The listing builds one solid part. Answer for the finished solid, in the listing's coordinates (mm). Coordinates: 2 decimals unless noted, no trailing zeros. Loops run counter-clockwise (first coordinate to the right, second up) from the corner with the lowest first, then second, coordinate; pieces in that order, holes last. Notation, with made-up numbers: M 17,-10.5 L 44,-10.5 A16 cw 44,0.5 Z; hole C 19.25,-8.5 d9. An arc over 180 degrees is marked long. Return JSON: item names as keys, results as strings. Group by question number.
1. Straight lines are drawn through the part: L1, parallel to Z at x = 209.5, y = -2.75; L2, parallel to Y at x = 290, z = -7.2. For each, find the intervals that lie inside material, in ascending order. Write a range as from..to.
2. Given P1, Ø3.5, axis at x = 290, y = 0, coming from the +Z side; P2, Ø4, axis at x = 20, y = 0, coming from the -Z side, each flat-ended and moving along its own axis, determine where each tip first touches the part or whether it passes through.
3. Section B-B (z = 1.5) is taken. Write down the section's boundary in (x, y), then the cut area to 3 significant figures.
4. Section A-A (x = 164) is taken. Write down the section's boundary in (y, z), then the cut area to 3 significant figures.
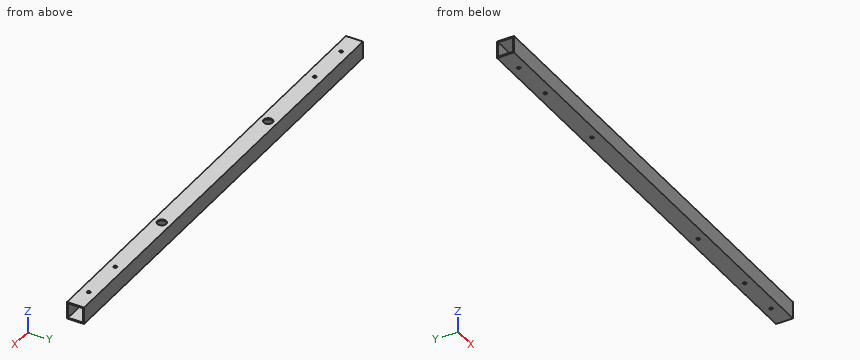
```python
from build123d import *

# Parameters (mm, degrees)
SKETCH_1_W          = 15
SKETCH_1_H          = 15
SKETCH_1_W_2        = 13
SKETCH_1_H_2        = 13
EXTRUDE_1_DEPTH     = 420
SKETCH_2_R          = 1.5
CUT_EXTRUDE_1_DEPTH = 421.334688076
SKETCH_3_R          = 4
CUT_EXTRUDE_2_DEPTH = 10


with BuildPart() as part:
    # 草图1 → 凸台-拉伸1 (new body)
    with BuildSketch(Plane(origin=(0, 0, 0), x_dir=(0, 0, -1), z_dir=(1, 0, 0))):
        Rectangle(SKETCH_1_W, SKETCH_1_H)
        Rectangle(SKETCH_1_W_2, SKETCH_1_H_2, mode=Mode.SUBTRACT)
    extrude(amount=EXTRUDE_1_DEPTH)

    # 草图2 → 切除-拉伸1 (cut, through all)
    with BuildSketch(Plane.XY.offset(7.5)):
        with Locations((20, 0)):
            Circle(SKETCH_2_R)
        with Locations((60, 0)):
            Circle(SKETCH_2_R)
        with Locations((130, 0)):
            Circle(SKETCH_2_R)
        with Locations(Location((290, 0, 0), (0, 0, 270))):
            Circle(SKETCH_2_R)
        with Locations(Location((360, 0, 0), (0, 0, 270))):
            Circle(SKETCH_2_R)
        with Locations(Location((400, 0, 0), (0, 0, 270))):
            Circle(SKETCH_2_R)
    extrude(amount=-CUT_EXTRUDE_1_DEPTH, mode=Mode.SUBTRACT)

    # 草图3 → 切除-拉伸2 (cut)
    with BuildSketch(Plane.XY.offset(7.5)):
        with Locations((130, 0)):
            Circle(SKETCH_3_R)
        with Locations((290, 0)):
            Circle(SKETCH_3_R)
    extrude(amount=-CUT_EXTRUDE_2_DEPTH, mode=Mode.SUBTRACT)


solid = part.part
```
Worked out:
{
 "1": {"L1": "-7.5..-6.5, 6.5..7.5", "L2": "-7.5..-1.5, 1.5..7.5"},
 "2": {"P1": "z = -6.5", "P2": "z = -7.5"},
 "3": {"outline": "M 0,-7.5 L 420,-7.5 L 420,-6.5 L 0,-6.5 Z; M 0,6.5 L 420,6.5 L 420,7.5 L 0,7.5 Z", "area": "840 mm^2"},
 "4": {"outline": "M -7.5,-7.5 L 7.5,-7.5 L 7.5,7.5 L -7.5,7.5 Z; hole M -6.5,-6.5 L 6.5,-6.5 L 6.5,6.5 L -6.5,6.5 Z", "area": "56.0 mm^2"}
}
